```python
from build123d import *

# Parameters (mm, degrees)
SKETCH1_W           = 24
SKETCH1_H           = 88
BOSS_EXTRUDE1_DEPTH = 1.2
BOSS_EXTRUDE2_START = 7.5
SKETCH2_R           = 2
BOSS_EXTRUDE2_DEPTH = 36.5
SKETCH4_R           = 2.25
CUT_EXTRUDE2_DEPTH  = 49.276702456


with BuildPart() as part:
    # Sketch1 → Boss-Extrude1 (new body)
    with BuildSketch(Plane(origin=(0, 0, 0), x_dir=(1, 0, 0), z_dir=(0, 1, 0))):
        Rectangle(SKETCH1_W, SKETCH1_H)
    extrude(amount=BOSS_EXTRUDE1_DEPTH)

    # Sketch2 → Boss-Extrude2 (add)
    with BuildSketch(Plane.XY.offset(BOSS_EXTRUDE2_START)):
        with BuildLine():
            Line((-12, 0), (-15.5, 0))
            ThreePointArc((-15.5, 0), (-16.949137675, 6.685906464), (-12.861818808, 1.2))
            Line((-12.861818808, 1.2), (-12, 1.2))
            Line((-12, 1.2), (-12, 0))
        make_face()
        with Locations(Location((-15.5, 3.5, 0), (0, 0, 180))):
            Circle(SKETCH2_R, mode=Mode.SUBTRACT)
    extrude(amount=BOSS_EXTRUDE2_DEPTH)

    # Mirror4: part across plane


with BuildPart() as part_1:
    add(part.part)
    add(part.part.mirror(Plane.XY))

    # Sketch4 → Cut-Extrude2 (cut, through all)
    with BuildSketch(Plane(origin=(0, 1.2, 0), x_dir=(1, 0, 0), z_dir=(0, 1, 0))):
        with Locations(Location((1.5, 34, 0), (0, 0, 270))):
            Circle(SKETCH4_R)
        with Locations(Location((1.5, -34, 0), (0, 0, 90))):
            Circle(SKETCH4_R)
    extrude(amount=-CUT_EXTRUDE2_DEPTH, mode=Mode.SUBTRACT)


solid = part_1.part
```
CAD build for the part. Positions are in the model's coordinates, mm. A direction names the side the tool comes from. Give positions to 0.01 mm unless a question says otherwise; leave off trailing zeros. Loops run counter-clockwise (first coordinate to the right, second up) from the corner with the lowest first, then second, coordinate; pieces in that order, holes last. Notation, with made-up numbers: (36, -3.75) - (45, -3.75) arc R21 ccw to (45, 10.25) - close; hole circle Ø4 at (31.5, 88.5). An arc over 180 degrees is marked (long way). Put each result on its own line as item: value.
Q1. Tool access for faces 1 (the face through (-13.9, 2, 7.5)), 2 (the face through (-2, 0, 1)): list every direction of +Z, -Z, +X, -X, +Y, -Y with a clear straight run to the whole face (end or side of a thin tool).
Filled in:
face 1: -X, +Y, -Y
face 2: +Z, -Z, +X, -X, -Y
Q2. Slice it at D-D (z = -4). Give the cut face in (x, y), plus the area to 3 significant figures.
Filled in:
outline: (-12, 0) - (12, 0) - (12, 1.2) - (-12, 1.2) - close
area: 28.8 mm²
Q3. Slice it at A-A (z = 34). Give the cut face in (x, y), plus the area to 3 significant figures.
Filled in:
outline: (-15.5, 0) - (-0.75, 0) - (-0.75, 1.2) - (-12.86, 1.2) arc R3.5 ccw (long way) to start; (3.75, 0) - (12, 0) - (12, 1.2) - (3.75, 1.2) - close; hole circle Ø4 at (-15.5, 3.5)
area: 51.3 mm²
Q4. Flat gauge pin, fed straight in: pin 1 (4 mm diameter, centred on x = 2.5, z = 2.5, fed in from +Y). Where does the tip first touch, or does it go through?
Filled in:
pin 1: stops at y = 1.2
Q5. Probe line 1 along Y through (x, z) = (-15.5, -32.5); line 2 along Y through (x, z) = (-10.5, -39.5); line 3 along Y through (x, z) = (-14, 25.5). List the from-to ranges inside material, lowest first.
Filled in:
line 1: y = 0 to 1.5, 5.5 to 7
line 2: y = 0 to 1.2
line 3: y = 0 to 2.18, 4.82 to 6.66
Q6. Slice it at C-C (z = -35). Give the cut face in (x, y).
Filled in:
outline: (-15.5, 0) - (-0.52, 0) - (-0.52, 1.2) - (-12.86, 1.2) arc R3.5 ccw (long way) to start; (3.52, 0) - (12, 0) - (12, 1.2) - (3.52, 1.2) - close; hole circle Ø4 at (-15.5, 3.5)
Q7. Mould opens along X. For faces 3 (the face through (-13.9, 4.7, -25.5)), 4 (the face through (-13.9, 2, -7.5)) say: pulls with the +X half, pulls with the -X half, needs draft (parallel to the pull), parting line crosses it, or undercut.
Filled in:
face 3: undercut
face 4: needs draft
Q8. Slice it at B-B (y = 3.5). Give the cut face in (x, z), plus the area to 3 significant figures.
Filled in:
outline: (-19, -44) - (-17.5, -44) - (-17.5, -7.5) - (-19, -7.5) - close; (-19, 7.5) - (-17.5, 7.5) - (-17.5, 44) - (-19, 44) - close; (-13.5, -44) - (-12, -44) - (-12, -7.5) - (-13.5, -7.5) - close; (-13.5, 7.5) - (-12, 7.5) - (-12, 44) - (-13.5, 44) - close
area: 219 mm²
